```python
from build123d import *

# Parameters (mm, degrees)
SKETCH1_W           = 80
SKETCH1_H           = 80
BOSS_EXTRUDE1_DEPTH = 3.175
SKETCH3_OUTSIDE_W   = 104.636
SKETCH3_OUTSIDE_H   = 104.636
CUT_EXTRUDE1_DEPTH  = 57.657573413


with BuildPart() as part:
    # Sketch1 → Boss-Extrude1 (new body)
    with BuildSketch(Plane(origin=(0, 0, 0), x_dir=(1, 0, 0), z_dir=(0, 1, 0))):
        Rectangle(SKETCH1_W, SKETCH1_H)
    extrude(amount=BOSS_EXTRUDE1_DEPTH)

    # Sketch3 outside → Cut-Extrude1 (cut, through all)
    with BuildSketch(Plane(origin=(0, 3.175, 0), x_dir=(1, 0, 0), z_dir=(0, 1, 0))):
        Rectangle(SKETCH3_OUTSIDE_W, SKETCH3_OUTSIDE_H)
        Polygon((-40, -40), (-34.666666667, -40), (-34.666666667, -36.825), (-29.333333333, -36.825), (-29.333333333, -40), (-24, -40), (-24, -36.825), (-18.666666667, -36.825), (-18.666666667, -40), (-13.333333333, -40), (-13.333333333, -36.825), (-8, -36.825), (-8, -40), (-2.666666667, -40), (-2.666666667, -36.825), (2.666666667, -36.825), (2.666666667, -40), (8, -40), (8, -36.825), (13.333333333, -36.825), (13.333333333, -40), (18.666666667, -40), (18.666666667, -36.825), (24, -36.825), (24, -40), (29.333333333, -40), (29.333333333, -36.825), (34.666666667, -36.825), (34.666666667, -40), (40, -40), (40, -34.666666667), (36.613333333, -34.666666667), (36.613333333, -29.333333333), (40, -29.333333333), (40, -24), (36.613333333, -24), (36.613333333, -18.666666667), (40, -18.666666667), (40, -13.333333333), (36.613333333, -13.333333333), (36.613333333, -8), (40, -8), (40, -2.666666667), (36.613333333, -2.666666667), (36.613333333, 2.666666667), (40, 2.666666667), (40, 8), (36.613333333, 8), (36.613333333, 13.333333333), (40, 13.333333333), (40, 18.666666667), (36.613333333, 18.666666667), (36.613333333, 24), (40, 24), (40, 29.333333333), (36.613333333, 29.333333333), (36.613333333, 34.666666667), (40, 34.666666667), (40, 40), (34.666666667, 40), (34.666666667, 36.825), (29.333333333, 36.825), (29.333333333, 40), (24, 40), (24, 36.825), (18.666666667, 36.825), (18.666666667, 40), (13.333333333, 40), (13.333333333, 36.825), (8, 36.825), (8, 40), (2.666666667, 40), (2.666666667, 36.825), (-2.666666667, 36.825), (-2.666666667, 40), (-8, 40), (-8, 36.825), (-13.333333333, 36.825), (-13.333333333, 40), (-18.666666667, 40), (-18.666666667, 36.825), (-24, 36.825), (-24, 40), (-29.333333333, 40), (-29.333333333, 36.825), (-34.666666667, 36.825), (-34.666666667, 40), (-40, 40), (-40, 34.666666667), (-36.613333333, 34.666666667), (-36.613333333, 29.333333333), (-40, 29.333333333), (-40, 24), (-36.613333333, 24), (-36.613333333, 18.666666667), (-40, 18.666666667), (-40, 13.333333333), (-36.613333333, 13.333333333), (-36.613333333, 8), (-40, 8), (-40, 2.666666667), (-36.613333333, 2.666666667), (-36.613333333, -2.666666667), (-40, -2.666666667), (-40, -8), (-36.613333333, -8), (-36.613333333, -13.333333333), (-40, -13.333333333), (-40, -18.666666667), (-36.613333333, -18.666666667), (-36.613333333, -24), (-40, -24), (-40, -29.333333333), (-36.613333333, -29.333333333), (-36.613333333, -34.666666667), (-40, -34.666666667), align=None, mode=Mode.SUBTRACT)
    extrude(amount=-CUT_EXTRUDE1_DEPTH, mode=Mode.SUBTRACT)


solid = part.part
```
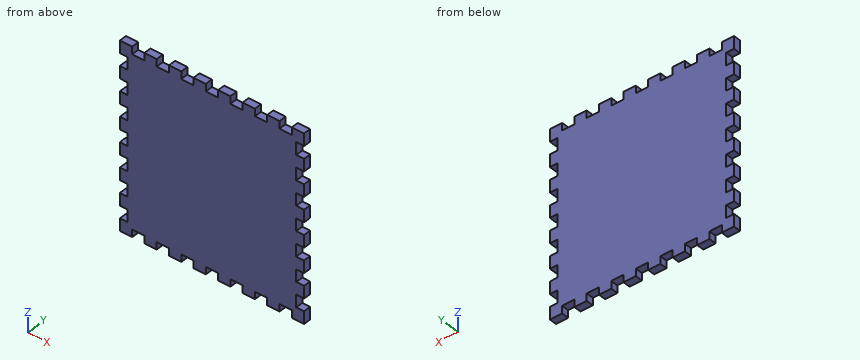
Work out the finished part from the listing and answer in its coordinate system (mm). Round coordinates to 2 decimals unless told otherwise and drop trailing zeros. Write each loop counter-clockwise with the first axis right and the second up, starting at its lowest first coordinate (ties: lowest second). Pieces come first, ordered by that corner, then holes.
1) A cutting plane is placed at A-A on x = 32. Determine the outline of the cut face in (y, z) (3 decimals), and give its area (3 significant figures).
2) Consider probe 1 along X at (y, z) = (1.2, 13); probe 2 along Z at (x, y) = (33.5, 1.4) (3 decimals). Determine where each line is inside the solid, lowest interval first.
3) A cutting plane is placed at B-B on z = 11. Determine the outline of the cut face in (x, y) (3 decimals), and give its area (3 significant figures).
4) Flat-ended cylindrical pins translate along their axes: P1, Ø1.5, axis at y = 2.5, z = 20, coming from the +X side; P2, Ø1, axis at x = 22, y = 2, coming from the -Z side (3 decimals). Find the tip coordinate at first contact, or state that the pin passes through.
Entries:
1. outline: (0, -36.825) - (3.175, -36.825) - (3.175, 36.825) - (0, 36.825) - close
1. area: 234 mm2
2. probe 1: x = -36.61 to 36.61
2. probe 2: z = -36.825 to 36.825
3. outline: (-36.613, 0) - (36.613, 0) - (36.613, 3.175) - (-36.613, 3.175) - close
3. area: 232 mm2
4. P1: stops at x = 36.61
4. P2: stops at z = -36.825
